```python
from build123d import *

# Parameters (mm, degrees)
SKETCH_1_R          = 1.1
EXTRUDE_1_DEPTH     = 9
EXTRUDE_2_DEPTH     = 2
EXTRUDE_3_DEPTH     = 3.5
CUT_EXTRUDE_1_DEPTH = 3


with BuildPart() as part:
    # 草图1 → 凸台-拉伸1 (new body)
    with BuildSketch(Plane(origin=(0, 0, 0), x_dir=(0, 0, -1), z_dir=(1, 0, 0))):
        with BuildLine():
            Line((-44.956504104, -32.544780514), (-40.285971637, -28.762657896))
            ThreePointArc((-40.285971637, -28.762657896), (-36.785668861, -33.121965015), (-32.816123753, -37.05876444))
            Line((-32.816123753, -37.05876444), (-37.065731089, -41.308371776))
            ThreePointArc((-37.065731089, -41.308371776), (-41.244537814, -37.136748653), (-44.956504104, -32.544780514))
        make_face()
        with Locations((-40.800162976, -33.03932053)):
            Circle(SKETCH_1_R, mode=Mode.SUBTRACT)
        with Locations((-37.123106012, -37.123106012)):
            Circle(SKETCH_1_R, mode=Mode.SUBTRACT)
    extrude(amount=EXTRUDE_1_DEPTH)

    # 草图2 → 凸台-拉伸2 (add)
    with BuildSketch(Plane.ZY):
        with BuildLine():
            Line((42.469798969, -35.729066257), (47.254371389, -44.844869924))
            Line((47.254371389, -44.844869924), (44.155307417, -46.47146222))
            Line((44.155307417, -46.47146222), (39.972641515, -38.502440576))
            ThreePointArc((39.972641515, -38.502440576), (41.244537814, -37.136748653), (42.469798969, -35.729066257))
        make_face()
    extrude(amount=-EXTRUDE_2_DEPTH)

    # 草图3 → 凸台-拉伸3 (add)
    with BuildSketch(Plane(origin=(0, 9.759553772, 18.594383834), x_dir=(1, 0, 0), z_dir=(0, 0.4647406558327103, 0.8854468492327375))):
        Polygon((2, -51.373631369), (2, -54.373631369), (9, -51.373631369), align=None)
    extrude(amount=-EXTRUDE_3_DEPTH)

    # 草图4 → 切除-拉伸1 (cut)
    with BuildSketch(Plane.ZY):
        with BuildLine():
            Line((40.800162976, -30.93932053), (42.621237871, -30.653719205))
            Line((42.621237871, -30.653719205), (44.956504104, -32.544780514))
            ThreePointArc((44.956504104, -32.544780514), (43.74213685, -34.159558894), (42.469798969, -35.729066257))
            Line((42.469798969, -35.729066257), (40.199666496, -35.051633621))
            ThreePointArc((40.199666496, -35.051633621), (38.722200333, -32.735888076), (40.800162976, -30.93932053))
        make_face()
        with BuildLine():
            Line((34.940927421, -39.183568108), (35.023106012, -37.123106012))
            ThreePointArc((35.023106012, -37.123106012), (36.71133724, -35.063871573), (39.061626467, -36.315555119))
            Line((39.061626467, -36.315555119), (39.972641515, -38.502440576))
            ThreePointArc((39.972641515, -38.502440576), (38.544727601, -39.93186665), (37.065731089, -41.308371776))
            Line((37.065731089, -41.308371776), (34.940927421, -39.183568108))
        make_face()
    extrude(amount=-CUT_EXTRUDE_1_DEPTH, mode=Mode.SUBTRACT)


solid = part.part
```
The model under review builds one solid part; all positions refer to its coordinate system, in mm. A direction names the side the tool comes from. Coordinates: 2 decimals unless noted, no trailing zeros. Order: outer loops, then holes, each group sorted by start corner. A loop starts at its lowest first (then second) coordinate and runs counter-clockwise, first axis right, second up. Notation, with made-up numbers: (20.25, 39.5) -> (44.25, 39.5) arc R30 ccw to (44.25, 62.5) -> close; hole circle Ø6 at (37.5, 20.25). An arc over 180 degrees is marked (long way). Answer in a Markdown table with one row per item. Add a question column.
Item 1: We need section B-B on z = 37.5. Write out the cut boundary in (x, y), plus the area to 3 significant figures.
Item 2: Clearance check with flat-ended pins moving along their axes: pin 1 (2 mm diameter, centred on y = -38.5, z = 36, fed in from -X); pin 2 (4 mm diameter, centred on y = -42.5, z = 45.5, fed in from +X); pin 3 (3 mm diameter, centred on y = -37.12, z = 37.12, fed in from +X); pin 4 (4 mm diameter, centred on x = 3, z = 45, fed in from +Y). State where each tip first meets the part, or that it passes through.
Item 3: Mouldability with a two-part tool opening along Z and no side actions: class faces 1 (the flat face through (2, -42, 44)), 2 (the flat face through (1.48, -37.39, 39.51)), 3 (the flat face through (1.5, -30.8, 41.7)) as +Z half, -Z half, draft (parallel to the pull), parting line (faces both ways), or undercut.
Item 4: We need section D-D on x = 3.5. Write out the cut boundary in (y, z), plus the area to 3 significant figures.
Item 5: Machinability: for faces 4 (the cylindrical face through (5.958, -34.182, 43.725)), 5 (the flat face through (1.48, -38.17, 34.98)), 6 (the cylindrical face through (4.44, -33.06, 36.84)), 7 (the cylindrical face through (1.479, -32.777, 38.717)), which of the approach directions +Z, -Z, +X, -X, +Y, -Y give a long, thin tool a straight path to every point of the face, cutting with its end or side? Answer none if there is none.
Item 6: To check wall thickness, follow probe 1 along X at (y, z) = (-38, 35.5); probe 2 along Y at (x, z) = (4, 40.25); probe 3 along Z at (x, y) = (2.5, -37). State the ranges of each line that lie inside material, in increasing order.
Item 7: We need section A-A on x = 1. Write out the cut boundary in (y, z), plus the area to 3 significant figures.
Item 8: We need section C-C on y = -39.5. Write out the cut boundary in (x, z).
Final values:
| question | item | result |
|---|---|---|
| 1 | outline | (0, -35.06) -> (3, -35.06) -> (3, -36.09) -> (9, -36.09) -> (9, -32.31) -> (0, -32.31) -> close; (3, -40.91) -> (9, -40.91) -> (9, -38.16) -> (3, -38.16) -> close |
| 1 | area | 47.5 mm2 |
| 2 | pin 1 | stops at x = 3 |
| 2 | pin 2 | stops at x = 2 |
| 2 | pin 3 | stops at x = 9 |
| 2 | pin 4 | stops at y = -30.96 |
| 3 | face 1 | draft |
| 3 | face 2 | undercut |
| 3 | face 3 | +Z half |
| 4 | outline | (-41.31, 37.07) -> (-37.06, 32.82) arc R49.5 cw to (-28.76, 40.29) -> (-32.54, 44.96) arc R55.5 ccw to (-35.73, 42.47) -> (-37.82, 43.57) -> (-39.44, 40.47) -> (-38.5, 39.97) arc R55.5 ccw to start; hole circle Ø2.2 at (-37.12, 37.12); hole circle Ø2.2 at (-33.04, 40.8) |
| 4 | area | 67.3 mm2 |
| 5 | face 4 | +Z, +X, -X |
| 5 | face 5 | -X, -Y |
| 5 | face 6 | -Z, +X, -X, +Y |
| 5 | face 7 | +Z, -X |
| 6 | probe 1 | x = 3 to 9 |
| 6 | probe 2 | y = -39.03 to -33.99, -32.09 to -28.81 |
| 6 | probe 3 | z = 32.88 to 35.03, 39.35 to 43.14 |
| 7 | outline | (-46.47, 44.16) -> (-38.5, 39.97) -> (-36.32, 39.06) arc R2.1 cw to (-37.12, 35.02) -> (-39.18, 34.94) -> (-37.06, 32.82) arc R49.5 cw to (-28.76, 40.29) -> (-30.65, 42.62) -> (-30.94, 40.8) arc R2.1 cw to (-35.05, 40.2) -> (-35.73, 42.47) -> (-44.84, 47.25) -> close |
| 7 | area | 60.1 mm2 |
| 8 | outline | (0, 40.5) -> (3.35, 40.5) -> (2, 41.74) -> (2, 44.45) -> (0, 44.45) -> close; (3, 35.26) -> (9, 35.26) -> (9, 38.99) -> (3, 38.99) -> close |
